Model file for the job. Use its own axes, mm. A direction names the side the tool comes from. Coordinates: 2 decimals unless noted, no trailing zeros. Loops run counter-clockwise (first coordinate to the right, second up) from the corner with the lowest first, then second, coordinate; pieces in that order, holes last. Notation, with made-up numbers: (-19.75, 35) -> (-1.75, 35) arc R15 ccw to (-1.75, 44) -> close; hole circle Ø6 at (84.5, -21.75). An arc over 180 degrees is marked (long way). Use one line per item in the form item = value.
```python
from build123d import *

# Parameters (mm, degrees)
ESQUISSE1_W       = 40
ESQUISSE1_H       = 38
EXTRUSION1_DEPTH  = 19
ESQUISSE2_R       = 6
EXTRUSION2_DEPTH  = 1.5
ESQUISSE3_R       = 2.5
EXTRUSION3_DEPTH  = 3.5
D_ME1_FACE_RADIUS = 2.5
D_ME1_HEIGHT      = 1


with BuildPart() as part:
    # Esquisse1 → Extrusion1 (new body)
    with BuildSketch(Plane(origin=(0, 0, 0), x_dir=(0, 0, -1), z_dir=(1, 0, 0))):
        with Locations((-4.8337322, -1.663178935)):
            Rectangle(ESQUISSE1_W, ESQUISSE1_H)
    extrude(amount=EXTRUSION1_DEPTH)

    # Esquisse2 → Extrusion2 (add)
    with BuildSketch(Plane(origin=(0, 17.336821065, 0), x_dir=(1, 0, 0), z_dir=(0, 1, 0))):
        with Locations(Location((9, -14.8337322, 0), (0, 0, 90))):
            Circle(ESQUISSE2_R)
    extrude(amount=EXTRUSION2_DEPTH)

    # Esquisse3 → Extrusion3 (add)
    with BuildSketch(Plane(origin=(0, 18.836821065, 0), x_dir=(-1, 0, 0), z_dir=(0, 1, 0))):
        with Locations(Location((-10, 14.8337322, 0), (0, 0, 90))):
            Circle(ESQUISSE3_R)
    extrude(amount=EXTRUSION3_DEPTH)

    # Dôme1: a dome of height H over a round flat face of radius A is a cap of a sphere of radius (A * A + H * H) / (2 * H)
    d_me1_r = (D_ME1_FACE_RADIUS * D_ME1_FACE_RADIUS + D_ME1_HEIGHT * D_ME1_HEIGHT) / (2 * D_ME1_HEIGHT)
    d_me1_base = Plane((10, 22.336821065, 14.8337322), z_dir=(0, 1, 0))
    with Locations(d_me1_base.offset(D_ME1_HEIGHT - d_me1_r)):
        d_me1_ball = Sphere(d_me1_r, mode=Mode.PRIVATE)
    add(split(d_me1_ball, bisect_by=d_me1_base, keep=Keep.TOP, mode=Mode.PRIVATE))


solid = part.part
```
Q1. Which spindle directions (+Z, -Z, +X, -X, +Y, -Y) get a long thin tool onto all of the face, cutting with end or side? Do faces 1 (the face through (12.651, 18.076, 19.595)), 2 (the face through (9, -2, -15.166)). Say none if no direction does.
Result:
face_1 = +Y
face_2 = -Z, +X, -X, +Y, -Y
Q2. Wall check: line 1 along Y through (x, z) = (3.5, 15); line 2 along Y through (x, z) = (6.75, -5.5); line 3 along Z through (x, y) = (14, 18). Give the ranges that are in metal, low to high.
Result:
line_1 = -20.66 to 18.84
line_2 = -20.66 to 17.34
line_3 = 11.52 to 18.15
Q3. Band-saw the part on C-C, the plane x = 13. Write the cut outline in (y, z), and give its area (3 significant figures).
Result:
outline = (-20.66, -15.17) -> (17.34, -15.17) -> (17.34, 10.36) -> (18.84, 10.36) -> (18.84, 19.31) -> (17.34, 19.31) -> (17.34, 24.83) -> (-20.66, 24.83) -> close
area = 1,530 mm2
Q4. Band-saw the part on A-A, the plane x = 10. Write the cut outline in (y, z) (3 decimals), and give its area (3 significant figures).
Result:
outline = (-20.663, -15.166) -> (17.337, -15.166) -> (17.337, 8.918) -> (18.837, 8.918) -> (18.837, 12.334) -> (22.337, 12.334) arc R3.625 ccw to (22.337, 17.334) -> (18.837, 17.334) -> (18.837, 20.75) -> (17.337, 20.75) -> (17.337, 24.834) -> (-20.663, 24.834) -> close
area = 1,560 mm2
Q5. Band-saw the part on D-D, the plane x = 17.5. Write the cut outline in (y, z).
Result:
outline = (-20.66, -15.17) -> (17.34, -15.17) -> (17.34, 24.83) -> (-20.66, 24.83) -> close
Q6. Pin check, flat tips, straight feed: pin 1 Ø3.5 at (x, z) = (9.5, 17.5) entering from +Y; pin 2 Ø9.5 at (x, z) = (8.5, 10) entering from +Y. Stop position of each tip, or through.
Result:
pin_1 = 23.21
pin_2 = 23.32
Q7. Band-saw the part on B-B, the plane z = 10.5. Write the cut outline in (x, y).
Result:
outline = (0, -20.66) -> (19, -20.66) -> (19, 17.34) -> (13.15, 17.34) -> (13.15, 18.84) -> (4.85, 18.84) -> (4.85, 17.34) -> (0, 17.34) -> close
